Source: CAD feature listing. Evaluate the final solid. Frame: model axes, mm. Give positions to 0.01 mm unless a question says otherwise; leave off trailing zeros. Order: outer loops, then holes, each group sorted by start corner. A loop starts at its lowest first (then second) coordinate and runs counter-clockwise, first axis right, second up.
```python
from build123d import *

# Parameters (mm, degrees)
F0_R     = 12.5
F0_R_2   = 10.5
F1_DEPTH = 80
F3_DEPTH = 12.5
F5_DEPTH = 25


with BuildPart() as f1:
    # F0 (on Front) → F1 (new body)
    with BuildSketch(Plane.XZ):
        Circle(F0_R)
        Circle(F0_R_2, mode=Mode.SUBTRACT)
    extrude(amount=F1_DEPTH)

    # F2 (on Top) → F3 (cut, symmetric)
    with BuildSketch(Plane.XY):
        Polygon((12.505536, -55.04792), (-12.494464, -80.04792), (12.505536, -80.04792), align=None)
    extrude(amount=F3_DEPTH, both=True, mode=Mode.SUBTRACT)

    # F4 (on Top) → F5 (cut, symmetric)
    with BuildSketch(Plane.XY):
        with BuildLine():
            Line((8.606103, 0), (-8.96935, 0))
            ThreePointArc((-8.96935, 0), (-0.181624, -2.84369), (8.606103, 0))
        make_face()
    extrude(amount=F5_DEPTH, both=True, mode=Mode.SUBTRACT)


solid = f1.part
```
1) Material intervals for L1, parallel to X at y = -44.5, z = 0; L2, parallel to Z at x = -7, y = -73, sorted ascending.
Report:
L1: x = -12.5 to -10.5, 10.5 to 12.5
L2: z = -10.36 to -7.83, 7.83 to 10.36
2) Pin query (flat end, axial travel): pin 1 (8 mm diameter, centred on x = -1.5, z = -9, fed in from -Y); pin 2 (2 mm diameter, centred on x = 7.5, y = -49.5, fed in from +Z); pin 3 (1 mm diameter, centred on x = -9.5, z = -1, fed in from +Y); pin 4 (2 mm diameter, centred on y = -8, z = 1, fed in from -X). Return the tip coordinate at first contact, or that it passes through.
Report:
pin 1: stops at y = -73.05
pin 2: stops at z = 10.68
pin 3: passes through
pin 4: stops at x = -12.5
3) Section query D-D, the plane x = 4. Return the cut outline in (y, z), and give its area (3 significant figures).
Report:
outline: (-63.55, -11.84) - (-2.25, -11.84) - (-2.25, -9.71) - (-63.55, -9.71) - close; (-63.55, 9.71) - (-2.25, 9.71) - (-2.25, 11.84) - (-63.55, 11.84) - close
area: 262 mm2
4) Section query A-A, the plane z = 0. Return the cut outline in (x, y).
Report:
outline: (-12.5, -80) - (-12.45, -80) - (-10.5, -78.05) - (-10.5, 0) - (-12.5, 0) - close; (10.5, -57.05) - (12.5, -55.05) - (12.5, 0) - (10.5, 0) - close
5) Draft query along Z for faces 1 (the cylindrical face through (-10.49, -29.97, 0.46)), 2 (the flat face through (0.085, -67.469, -11.053)), 3 (the cylindrical face through (-12.488, -30.551, 0.55)). Return one class per face: +Z half, -Z half, draft (parallel to the pull), parting line (faces both ways), or undercut.
Report:
face 1: undercut
face 2: draft
face 3: parting line
6) Section query C-C, the plane y = -27. Return the cut outline in (x, z).
Report:
outline: circle Ø25 at (0, 0); hole circle Ø21 at (0, 0)
7) Section query B-B, the plane x = -7.5. Return the cut outline in (y, z).
Report:
outline: (-75.05, -10) - (-0.94, -10) - (-0.94, -7.35) - (-75.05, -7.35) - close; (-75.05, 7.35) - (-0.94, 7.35) - (-0.94, 10) - (-75.05, 10) - close
